from build123d import *

# Parameters (mm, degrees)
F0_R     = 20
F1_DEPTH = 5
F2_DEPTH = 3.5


with BuildPart() as f1:
    # F0 (on Top) → F1 (new body)
    with BuildSketch(Plane.XY):
        Polygon((9.999996, 9.999996), (440.000004, 9.999996), (440.000004, 340.000004), (109.999996, 340.000004), (109.999996, 240.000004), (9.999996, 240.000004), align=None)
        with Locations((60, 175)):
            Circle(F0_R, mode=Mode.SUBTRACT)
        with Locations((390, 175)):
            Circle(F0_R, mode=Mode.SUBTRACT)
    extrude(amount=F1_DEPTH)

    # F0 (on Top) → F2 (join)
    with BuildSketch(Plane.XY):
        Polygon((0, 250), (0, 0), (450, 0), (450, 350), (100, 350), (100, 250), align=None)
        Polygon((440.000004, 340.000004), (440.000004, 9.999996), (9.999996, 9.999996), (9.999996, 240.000004), (109.999996, 240.000004), (109.999996, 340.000004), align=None, mode=Mode.SUBTRACT)
    extrude(amount=F2_DEPTH)


solid = f1.part
Geometry: final body of the model. Coordinates: model frame, mm. Coordinates: 2 decimals unless noted, no trailing zeros. Loops run counter-clockwise (first coordinate to the right, second up) from the corner with the lowest first, then second, coordinate; pieces in that order, holes last. Notation, with made-up numbers: M 66,2 L 110,2 A33 cw 110,38 Z; hole C 46.5,43.25 d7. An arc over 180 degrees is marked long. One line per item, written item: value. Start each with the question number.
1) Draft query along Y for faces 1 (the cylindrical face through (70.752, 191.864, 2.465)), 2 (the flat face through (222, 177, 0)). Return one class per face: released by +Y, released by -Y, zero draft, split by the parting line, or undercut.
2) Material intervals for L1, parallel to Y at x = 390, z = 2.6; L2, parallel to X at y = 177, z = 0.7; L3, parallel to X at y = 129.5, z = 4.2, sorted ascending. Write a range as from..to.
3) Cut plane A-A (y = 175). Return loops of the section in (x, z).
4) Pin query (flat end, axial travel): P1, Ø1.2, axis at y = 196.5, z = 4.5, coming from the +X side; P2, Ø12, axis at x = 396.5, y = 249, coming from the -Z side; P3, Ø0.8, axis at y = 132, z = 4, coming from the -X side; P4, Ø0.8, axis at y = 283.5, z = 4.5, coming from the -X side. Return the tip coordinate at first contact, or that it passes through.
5) Cut plane D-D (x = 306). Return loops of the section in (y, z), then the cut area to 3 significant figures.
6) Cut plane B-B (x = 390). Return loops of the section in (y, z).
7) Cut plane C-C (y = 263). Return loops of the section in (x, z), then the cut area to 3 significant figures.
Evaluation:
1. face 1: undercut
1. face 2: zero draft
2. L1: 0..155, 195..350
2. L2: 0..40.1, 79.9..370.1, 409.9..450
2. L3: 10..440
3. outline: M 0,0 L 40,0 L 40,5 L 10,5 L 10,3.5 L 0,3.5 Z; M 80,0 L 370,0 L 370,5 L 80,5 Z; M 410,0 L 450,0 L 450,3.5 L 440,3.5 L 440,5 L 410,5 Z
4. P1: x = 440
4. P2: z = 0
4. P3: x = 10
4. P4: x = 110
5. outline: M 0,0 L 350,0 L 350,3.5 L 340,3.5 L 340,5 L 10,5 L 10,3.5 L 0,3.5 Z
5. area: 1,720 mm^2
6. outline: M 0,0 L 155,0 L 155,5 L 10,5 L 10,3.5 L 0,3.5 Z; M 195,0 L 350,0 L 350,3.5 L 340,3.5 L 340,5 L 195,5 Z
7. outline: M 100,0 L 450,0 L 450,3.5 L 440,3.5 L 440,5 L 110,5 L 110,3.5 L 100,3.5 Z
7. area: 1,720 mm^2
